Autodesk Inventor part; units mm, degrees
ref_plane "YZ Plane" through (0, 0, 0) normal (1, 0, 0) x (0, 1, 0)
ref_plane "XZ Plane" through (0, 0, 0) normal (0, 1, 0) x (-1, 0, 0)
ref_plane "XY Plane" through (0, 0, 0) normal (0, 0, 1) x (1, 0, 0)
sketch "Sketch1" plane through (0, 0, 0) normal (0, 1, 0) x (-1, 0, 0)
  line L0 (46.6228, 34.6302) -> (-74.0272, 34.6302)
  line L1 (-74.0272, 34.6302) -> (-74.0272, -28.8698)
  line L2 (-74.0272, -28.8698) -> (46.6228, -28.8698)
  line L3 (46.6228, -28.8698) -> (46.6228, 34.6302)
  point P0 (0, 0)
  dimension "d0" = 120.65
  dimension "d1" = 63.5
extrude "Extrusion1" add sketch "Sketch1" along normal blind 12.7
sketch "Sketch4" plane through (0, 0, 0) normal (0, -1, 0) x (1, 0, 0)
  line L0 (74.0272, -28.8698) -> (-46.6228, -28.8698)
  line L1 (-28.8428, 23.5502) -> (-28.8428, 29.5502)
  line L2 (-46.6228, -28.8698) -> (-46.6228, 34.6302)
  point P0 (0, 0)
  point P1 (-32.8428, -16.6898)
  point P2 (-32.8428, -23.7898)
  point P3 (-11.9428, -23.7898)
  point P4 (-11.9428, -16.6898)
  dimension "d21" = 0
  dimension "d22" = 0
  dimension "d23" = 0
  dimension "d24" = 0
  dimension "d25" = 5.08
  dimension "d26" = 7.1
  dimension "d27" = 20.9
  dimension "d35" = 4
  dimension "d92" = 13.78
hole "Hole2" at (-32.8428, 0, -16.6898) at (-32.8428, 0, -23.7898) at (-11.9428, 0, -23.7898) at (-11.9428, 0, -16.6898) direction (0, 1, 0) diameter 2.8 depth 25.4 tip angle 118
sketch "Sketch6" plane through (0, 0, 0) normal (0, -1, 0) x (1, 0, 0)
  line L0 (-46.6228, 34.6302) -> (74.0272, 34.6302)
  line L1 (-46.6228, -28.8698) -> (-46.6228, 34.6302)
  line L2 (74.0272, -28.8698) -> (-46.6228, -28.8698)
  point P0 (0, 0)
  point P1 (69.7092, -24.6788)
  point P2 (-42.0508, -24.6788)
  point P3 (-42.0508, 30.4392)
  point P4 (69.7092, 30.4392)
  dimension "d43" = 0
  dimension "d44" = 0
  dimension "d46" = 111.76
  dimension "d47" = 0
  dimension "d48" = 0
  dimension "d50" = 4.191
  dimension "d51" = 4.572
  dimension "d91" = 4.191
hole "Hole4" at (69.7092, 0, -24.6788) at (-42.0508, 0, -24.6788) at (-42.0508, 0, 30.4392) at (69.7092, 0, 30.4392) direction (0, 1, 0) diameter 4.8 depth 25.4 tip angle 118
sketch "Sketch10" plane through (0, 12.7, 0) normal (0, 1, 0) x (1, 0, 0)
  circle A0 centre (54.9772, -18.7552) radius 2.413
  circle A1 centre (4.1772, -18.7552) radius 2.413
  line L0 (74.0272, 28.8698) -> (-46.6228, 28.8698)
  point P0 (0, 0)
  point P1 (4.1772, 12.9948)
  point P2 (54.9772, 12.9948)
  point P3 (66.6772, 28.8698)
  point P4 (-45.6228, 28.8698)
  dimension "d80" = 0
  dimension "d81" = 0
  dimension "d82" = 0
  dimension "d83" = 15.875
hole "Hole7" at (4.1772, 12.7, -12.9948) at (54.9772, 12.7, -12.9948) direction (0, -1, 0) diameter 4.826 end through all countersink diameter 9.525 countersink angle 82
sketch "Sketch11" plane through (0, 0, 0) normal (0, -1, 0) x (1, 0, 0)
  line L0 (-28.8428, -3.0578) -> (-16.8428, -3.0578)
  line L1 (-16.8428, -3.0578) -> (-16.8428, -9.0578)
  line L2 (-16.8428, -9.0578) -> (-28.8428, -9.0578)
  line L3 (-28.8428, -9.0578) -> (-28.8428, -3.0578)
  line L4 (-28.8428, -17.7898) -> (-16.8428, -17.7898)
  line L5 (-16.8428, -17.7898) -> (-16.8428, -23.7898)
  line L6 (-16.8428, -23.7898) -> (-28.8428, -23.7898)
  line L7 (-28.8428, -23.7898) -> (-28.8428, -17.7898)
  line L8 (-28.8428, 23.5502) -> (-28.8428, 29.5502)
  line L9 (-16.8428, 29.5502) -> (-16.8428, 23.5502)
  line L10 (74.0272, -28.8698) -> (-46.6228, -28.8698)
  point P0 (0, 0)
  dimension "d93" = 0
  dimension "d94" = 0
  dimension "d95" = 0
  dimension "d96" = 0
  dimension "d97" = 6
  dimension "d98" = 6
  dimension "d99" = 5.08
  dimension "d100" = 19.812
extrude "Extrusion4" cut sketch "Sketch11" against normal blind 1.27
sketch "Sketch12" plane through (0, 0, 0) normal (0, -1, 0) x (1, 0, 0)
  circle A0 centre (-42.0508, 30.4392) radius 2.4
  circle A1 centre (69.7092, 30.4392) radius 2.4
  circle A2 centre (69.7092, -24.6788) radius 2.4
  circle A3 centre (-42.0508, -24.6788) radius 2.4
  point P0 (0, 0)
hole "Hole8" at (-42.0508, 0, 30.4392) at (69.7092, 0, 30.4392) at (69.7092, 0, -24.6788) at (-42.0508, 0, -24.6788) direction (0, 1, 0) diameter 4.826 end through all
sketch "Sketch13" plane through (0, 0, 0) normal (0, -1, 0) x (1, 0, 0)
  circle A0 centre (-32.8428, -16.6898) radius 1.4
  circle A1 centre (-32.8428, -23.7898) radius 1.4
  circle A2 centre (-11.9428, -16.6898) radius 1.4
  point P0 (0, 0)
  point P1 (-32.8428, -9.0698)
  point P2 (-32.8428, -1.9578)
  point P3 (-39.7887, 34.6302)
  point P4 (67.4471, 34.6302)
  point P5 (-11.9428, -9.0698)
  point P6 (-11.9428, -1.9578)
  dimension "d112" = 0
  dimension "d113" = 7.112
  dimension "d115" = 7.62
  dimension "d117" = 0
  dimension "d120" = 0
  dimension "d123" = 0
  dimension "d124" = 0
hole "Hole9" at (-32.8428, 0, -9.0698) at (-32.8428, 0, -1.9578) at (-11.9428, 0, -9.0698) at (-11.9428, 0, -1.9578) direction (0, 1, 0) diameter 2.8 end through all
sketch "Sketch15" plane through (0, 12.7, 0) normal (0, 1, 0) x (1, 0, 0)
  circle A0 centre (4.1772, -18.7552) radius 2.413
  circle A1 centre (54.9772, -18.7552) radius 2.413
  circle A2 centre (4.1772, -18.7552) radius 3.3734
  circle A3 centre (54.9772, -18.7552) radius 3.3734
  point P0 (0, 0)
  point P1 (4.1772, 12.9948)
  point P2 (54.9772, 12.9948)
  dimension "d140" = 6.7469
  dimension "d141" = 6.7469
extrude "Extrusion6" [suppressed]
sketch "Sketch16" plane through (0, 0, 0) normal (0, -1, 0) x (1, 0, 0)
  line L0 (-74.1492, 48.5934) -> (104.9801, 48.5934)
  line L1 (104.9801, 48.5934) -> (104.9801, 2.8802)
  line L2 (104.9801, 2.8802) -> (-74.1492, 2.8802)
  line L3 (-74.1492, 2.8802) -> (-74.1492, 48.5934)
  line L4 (-46.6228, 34.6302) -> (74.0272, 34.6302)
  point P0 (0, 0)
  dimension "d157" = 31.75
extrude "Extrusion7" cut sketch "Sketch16" against normal blind 25.4
sketch "Sketch17" plane through (0, 0, 0) normal (0, -1, 0) x (1, 0, 0)
  line L0 (74.0272, 2.8802) -> (-46.6228, 2.8802)
  line L1 (-46.6228, -28.8698) -> (-46.6228, 2.8802)
  line L2 (74.0272, -28.8698) -> (-46.6228, -28.8698)
  line L3 (74.0272, 2.8802) -> (74.0272, -28.8698)
  circle A0 centre (-11.9428, -9.0698) radius 1.4
  circle A1 centre (-32.8428, -9.0698) radius 1.4
  circle A2 centre (-32.8428, -1.9578) radius 1.4
  circle A3 centre (-11.9428, -1.9578) radius 1.4
  circle A4 centre (69.7092, -24.6788) radius 2.413
  circle A5 centre (-42.0508, -24.6788) radius 2.413
  line L4 (-28.8428, -9.0578) -> (-28.8428, -3.0578)
  line L5 (-28.8428, -3.0578) -> (-16.8428, -3.0578)
  line L6 (-16.8428, -3.0578) -> (-16.8428, -9.0578)
  line L7 (-16.8428, -9.0578) -> (-28.8428, -9.0578)
  line L8 (-28.8428, -23.7898) -> (-28.8428, -17.7898)
  line L9 (-28.8428, -17.7898) -> (-16.8428, -17.7898)
  line L10 (-16.8428, -17.7898) -> (-16.8428, -23.7898)
  line L11 (-16.8428, -23.7898) -> (-28.8428, -23.7898)
  circle A6 centre (4.1772, -12.9948) radius 2.413
  circle A7 centre (54.9772, -12.9948) radius 2.413
  circle A8 centre (-11.9428, -23.7898) radius 1.4
  circle A9 centre (-32.8428, -16.6898) radius 1.4
  circle A10 centre (-32.8428, -23.7898) radius 1.4
  circle A11 centre (-11.9428, -16.6898) radius 1.4
  circle A12 centre (-42.0508, -24.6788) radius 2.413
  point P0 (0, 0)
  point P1 (-42.0508, -2.1998)
  point P2 (69.7092, -2.1998)
  dimension "d146" = 0
  dimension "d147" = 0
  dimension "d148" = 0
  dimension "d149" = 5.08
hole "Hole10" at (-42.0508, 0, -2.1998) at (69.7092, 0, -2.1998) direction (0, 1, 0) diameter 3.9624 end through all
equation "\"d1\" = 2 * TalonSRXWidth"
equation "\"d28\" = CanConHoleDiam"
equation "\"d52\" = LegoMainHole"
equation "\"d125\" = CanConHoleDiam"
equation "\"LegoMainHole\" = 4.8"
equation "\"TalonSRXWidth\" = 31.75"
equation "\"TalonSRXFromSide\" = 15.875"
equation "\"TalonSRXBetweenHoles\" = 50.8"
equation "\"CanConPinWidth\" = 6"
equation "\"CanConPinLength\" = 12"
equation "\"CanConBetweenSideHoles\" = 20.9"
equation "\"CanConBetweenTopHoles\" = 7.1"
equation "\"CanConHoleDiam\" = 2.8"
equation "\"CanConHoleFromTopPin\" = 4"
properties part number "OneTalonSRXPlateTwo"
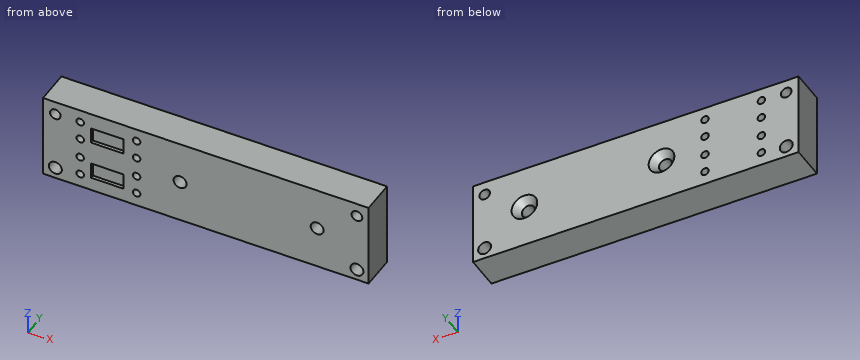
Design review of the part built by this model. Coordinates are the model's own, in mm. Coordinates: 2 decimals unless noted, no trailing zeros. Write each loop counter-clockwise with the first axis right and the second up, starting at its lowest first coordinate (ties: lowest second). Pieces come first, ordered by that corner, then holes. Notation, with made-up numbers: M 65.5,89 L 82.5,89 A22 ccw 82.5,117 Z; hole C 63.25,84 d8. An arc over 180 degrees is marked long. Answer as a JSON object with one key per item and string values.
Item 1: Insertion check: pin 1 Ø2.5 at (x, z) = (69.71, -2.2) entering from +Y. The pin has a flat end and moves straight along its axis. Give the tip position at first contact, or say it passes through.
Outcome:
{"pin 1": "through"}
Item 2: Add section A-A, the plane x = -27.5. Give the boundary of the cut face in (y, z), and give its area (3 significant figures).
Outcome:
{"outline": "M 0,-28.87 L 12.7,-28.87 L 12.7,2.88 L 0,2.88 L 0,-3.06 L 1.27,-3.06 L 1.27,-9.06 L 0,-9.06 L 0,-17.79 L 1.27,-17.79 L 1.27,-23.79 L 0,-23.79 Z", "area": "388 mm²"}
Item 3: Add section B-B, the plane y = 3. State how many separate pieces and enclosed holes the cut face has, and give its area (3 significant figures).
Outcome:
{"separate pieces": "1", "enclosed holes": "14", "area": "3,680 mm²"}
Item 4: Wall thickness on probe 1 along X at (y, z) = (10.25, -2); probe 2 along X at (y, z) = (7, -13); probe 3 along X at (y, z) = (4.5, -14.5): over which ranges is each line inside the solid? List them lowest first.
Outcome:
{"probe 1": "-46.62 to -44.02, -40.08 to -34.24, -31.44 to -13.34, -10.54 to 67.74, 71.68 to 74.03", "probe 2": "-46.62 to 1.76, 6.59 to 52.56, 57.39 to 74.03", "probe 3": "-46.62 to 2.29, 6.06 to 53.09, 56.86 to 74.03"}
